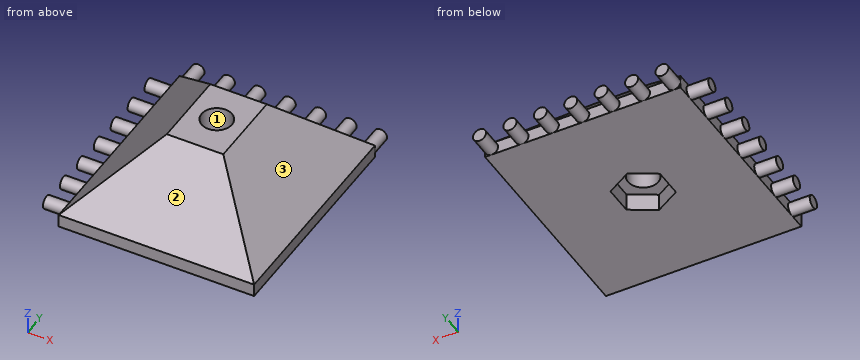
from build123d import *

# Parameters (mm, degrees)
SKETCH_W        = 45
SKETCH_H        = 50
PAD_DEPTH       = 25
CHAMFER_SIZE    = 22
SKETCH001_R     = 3.5
POCKET_DEPTH    = 25.001
SKETCH002_W     = 32.700705
SKETCH002_H     = 10
POCKET001_DEPTH = 45.001
SKETCH003_R     = 1.5
SKETCH003_R_2   = 1.518583
SKETCH003_R_3   = 1.500476
PAD001_DEPTH    = 5
SKETCH004_R     = 1.5
SKETCH004_R_2   = 1.504062
SKETCH004_R_3   = 1.509717
SKETCH004_R_4   = 1.483533
SKETCH004_R_5   = 1.504121
PAD002_DEPTH    = 5
POCKET002_DEPTH = 4


with BuildPart() as part:
    # Sketch → Pad (new body)
    with BuildSketch(Plane.XY):
        Rectangle(SKETCH_W, SKETCH_H)
    extrude(amount=PAD_DEPTH)

    # Chamfer
    chamfer_edges = [part.edges().sort_by_distance(p)[0] for p in [
        (0, 25, 25),
        (-22.5, 0, 25),
        (0, -25, 25),
        (22.5, 0, 25),
    ]]
    chamfer(chamfer_edges, length=CHAMFER_SIZE)

    # Sketch001 → Pocket (cut, through all)
    with BuildSketch(Plane(origin=(0, 0, 0), x_dir=(1, 0, 0), z_dir=(0, 0, -1))):
        Circle(SKETCH001_R)
    extrude(amount=-POCKET_DEPTH, mode=Mode.SUBTRACT)

    # Sketch002 → Pocket001 (cut, through all)
    with BuildSketch(Plane(origin=(-22.5, 0, 0), x_dir=(0, -1, 0), z_dir=(-1, 0, 0))):
        with Locations((-0.350352, 24)):
            Rectangle(SKETCH002_W, SKETCH002_H)
    extrude(amount=-POCKET001_DEPTH, mode=Mode.SUBTRACT)

    # Sketch003 → Pad001 (new body)
    with BuildSketch(Plane(origin=(0, 25, 0), x_dir=(-1, 0, 0), z_dir=(0, 1, 0))):
        with Locations((-21, 1.5)):
            Circle(SKETCH003_R)
        with Locations((-14, 1.5)):
            Circle(SKETCH003_R_2)
        with Locations((0, 1.5)):
            Circle(SKETCH003_R)
        with Locations((-7, 1.5)):
            Circle(SKETCH003_R)
        with Locations((7, 1.5)):
            Circle(SKETCH003_R_3)
        with Locations((14, 1.5)):
            Circle(SKETCH003_R)
        with Locations((21, 1.5)):
            Circle(SKETCH003_R)
    extrude(amount=PAD001_DEPTH)

    # Sketch004 → Pad002 (new body)
    with BuildSketch(Plane(origin=(-22.5, 0, 0), x_dir=(0, -1, 0), z_dir=(-1, 0, 0))):
        with Locations((0, 1.5)):
            Circle(SKETCH004_R)
        with Locations((-7, 1.5)):
            Circle(SKETCH004_R_2)
        with Locations((-14, 1.5)):
            Circle(SKETCH004_R)
        with Locations((-21, 1.5)):
            Circle(SKETCH004_R_3)
        with Locations((7, 1.5)):
            Circle(SKETCH004_R_4)
        with Locations((14, 1.5)):
            Circle(SKETCH004_R)
        with Locations((21, 1.5)):
            Circle(SKETCH004_R_5)
    extrude(amount=PAD002_DEPTH)

    # Sketch005 → Pocket002 (cut)
    with BuildSketch(Plane(origin=(0, 0, 0), x_dir=(1, 0, 0), z_dir=(0, 0, -1))):
        Polygon((5.7, -3.290897), (5.7, 3.290897), (0, 6.581793), (-5.7, 3.290897), (-5.7, -3.290897), (0, -6.581793), align=None)
    extrude(amount=-POCKET002_DEPTH, mode=Mode.SUBTRACT)


solid = part.part
Geometry: final body of the model. Coordinates: model frame, mm. Face numbers are marked on the shaded views. Round coordinates to 2 decimals unless told otherwise and drop trailing zeros. Loops run counter-clockwise (first coordinate to the right, second up) from the corner with the lowest first, then second, coordinate; pieces in that order, holes last. Notation, with made-up numbers: M 75.5,-38.75 L 81.5,-38.75 A21 ccw 81.5,-24.75 Z; hole C -19.5,13.5 d10. An arc over 180 degrees is marked long. Put each result on its own line as item: value. Start each with the question number.
(1) Section query C-C (y = -11). Return loops of the section in (x, z), then the cut area to 3 significant figures.
(2) Contact query for flat-ended pins moving along their axis: pin 1 Ø2.5 at (y, z) = (12, 1) entering from -X; pin 2 Ø0.9 at (y, z) = (24, 1) entering from -X; pin 3 Ø1.5 at (y, z) = (-13.5, 14.5) entering from -X; pin 4 Ø1.5 at (x, y) = (-6, -6) entering from -Z. Output: stop coordinate, or through.
(3) Section query B-B (z = 15.5). Return loops of the section in (x, y), then the cut area to 3 significant figures.
(4) Section query A-A (y = 26.5). Return loops of the section in (x, z).
(5) Draft query along Y for the marked faces 1, 2 and 3. Return one class per face: +Y half, -Y half, draft (parallel to the pull), parting line (faces both ways), or undercut.
(6) Material intervals for line 1 along X through (y, z) = (1, 11.5); line 2 along Y through (x, z) = (2.5, 15.75); line 3 along Y through (x, z) = (0, 14), sorted ascending. Write a range as [from, to].
(7) Section query D-D (x = 4.5). Return loops of the section in (y, z).
Findings below:
1. outline: M -22.5,0 L 22.5,0 L 22.5,3 L 8.5,17 L -8.5,17 L -22.5,3 Z
1. area: 569 mm2
2. pin 1: stops at x = -27.5
2. pin 2: stops at x = -22.5
2. pin 3: stops at x = -11.75
2. pin 4: stops at z = 0
3. outline: M -10,-12.5 L 10,-12.5 L 10,12.5 L -10,12.5 Z; hole C 0,0 d7
3. area: 462 mm2
4. outline: C -21,1.5 d3; C -14,1.5 d3; C -7,1.5 d3; C 0,1.5 d3; C 7,1.5 d3; C 14,1.5 d3.04; C 21,1.5 d3
5. face 1: undercut
5. face 2: -Y half
5. face 3: draft
6. line 1: x = [-14, -3.35], [3.35, 14]
6. line 2: y = [-12.25, -2.45], [2.45, 12.25]
6. line 3: y = [-14, -3.5], [3.5, 14]
7. outline: M -25,0 L -3.98,0 L -3.98,4 L 3.98,4 L 3.98,0 L 25,0 L 25,3 L 9,19 L -9,19 L -25,3 Z
